Autodesk Inventor part; units mm, degrees
ref_plane "YZ Plane" through (0, 0, 0) normal (1, 0, 0) x (0, 1, 0)
ref_plane "XZ Plane" through (0, 0, 0) normal (0, 1, 0) x (-1, 0, 0)
ref_plane "XY Plane" through (0, 0, 0) normal (0, 0, 1) x (1, 0, 0)
sketch "Sketch1" plane through (0, 0, 0) normal (0, 0, 1) x (1, 0, 0)
  line L0 (-25.5, 10) -> (25.5, 10)
  line L1 (25.5, 10) -> (25.5, -10)
  line L2 (25.5, -10) -> (-25.5, -10)
  line L3 (-25.5, -10) -> (-25.5, 10)
  point P0 (0, 0)
  point P1 (0, 10)
  point P2 (25.5, 0)
  dimension "d0" = 51
  dimension "d1" = 20
extrude "Extrusion1" add sketch "Sketch1" along normal blind 5
sketch "Sketch2" plane through (-25.5, -10, 0) normal (0, -1, 0) x (1, 0, 0)
  line L0 (0, 0) -> (51, 0)
  line L1 (10.5, 0) -> (10.5, -34)
  line L2 (10.5, -34) -> (15.5, -34)
  line L3 (15.5, -34) -> (15.5, 0)
  line L4 (35.5, 0) -> (35.5, -34)
  line L5 (35.5, -34) -> (40.5, -34)
  line L6 (40.5, -34) -> (40.5, 0)
  line L7 (15.5, -34) -> (35.5, -34) construction
  line L8 (0, 0) -> (10.5, -34)
  line L9 (4.1864, 0) -> (10.5, -20.444)
  line L10 (51, 0) -> (40.5, -34)
  line L11 (40.5, -20.444) -> (46.8136, 0)
  point P0 (25.5, 0)
  point P1 (25.5, 0)
  point P2 (25.5, -34)
  dimension "d4" = 20
  dimension "d5" = 5
  dimension "d6" = 5
  dimension "d7" = 34
  dimension "d8" = 4
  dimension "d9" = 4
extrude "Extrusion2" add sketch "Sketch2" against normal up to surface (20 mm away) contours L0 L6 L5 L4 | L0 L9 L1 L8 | L1 L0 L3 L2 | L0 L10 L6 L11
sketch "Sketch3" plane through (10, -10, -34) normal (-1, 0, 0) x (0, 0, 1)
  circle A0 centre (10, 10) radius 2.1
  line L0 (0, 0) -> (0, 20)
  point P0 (34, 10)
  point P1 (0, 10)
  dimension "d12" = 4.2
  dimension "d13" = 10
extrude "Extrusion3" cut sketch "Sketch3" along normal blind 40 and the other way blind 40
sketch "Sketch4" plane through (-25.5, 10, 5) normal (0, 1, 0) x (1, 0, 0)
  line L0 (35.5, 15) -> (15.5, 15)
  line L1 (15.5, 15) -> (15.5, 19)
  line L2 (15.5, 19) -> (35.5, 19)
  line L3 (35.5, 19) -> (35.5, 15)
  line L4 (10.5, 39) -> (15.5, 39)
  point P0 (25.5, 5)
  point P1 (35.5, 5)
  point P2 (15.5, 5)
  dimension "d18" = 20
  dimension "d19" = 4
extrude "Extrusion4" add sketch "Sketch4" against normal blind 5
sketch "Sketch6" plane through (0, 0, 5) normal (0, 0, 1) x (1, 0, 0)
  circle A0 centre (18, 0) radius 2.6
  circle A1 centre (-18, 0) radius 2.6
  point P0 (0, 0)
  dimension "d25" = 5.2
  dimension "d26" = 18
  dimension "d27" = 18
extrude "Extrusion6" cut sketch "Sketch6" against normal blind 5
properties part number "GT2_Holder"
CAD build for the part. Positions are in the model's coordinates, mm. A direction names the side the tool comes from. Round coordinates to 2 decimals unless told otherwise and drop trailing zeros. Loops run counter-clockwise (first coordinate to the right, second up) from the corner with the lowest first, then second, coordinate; pieces in that order, holes last. Notation, with made-up numbers: M 73,0 L 100,0 A24 ccw 100,27 Z; hole C 72,66 d10. An arc over 180 degrees is marked long. One line per question, with ' | ' between items. Start each with the question number.
Item 1: Two-plate mould, pull along Z, no slides. Class faces 4 (the cylindrical face through (20.48, 0.78, 2.54)), 5 (the flat face through (20.324, -0.14, -16.762)), 6 (the flat face through (-18.2, -0.14, -10.08)): pulls with the +Z half, pulls with the -Z half, needs draft (parallel to the pull), parting line crosses it, or undercut.
Item 2: Cut at D-D, the plane x = -20. Write the cut outline in (y, z).
Item 3: Which spindle directions (+Z, -Z, +X, -X, +Y, -Y) get a long thin tool onto all of the face, cutting with end or side? Do faces 1 (the flat face through (18.1, -0.1, -10.4)), 2 (the flat face through (0, 5, -12)), 3 (the cylindrical face through (-15.52, 0.78, 2.54)). Say none if no direction does.
Item 4: Cut at C-C, the plane z = -12.5. Write the cut outline in (x, y).
Item 5: Cut at B-B, the plane x = 17. Write the cut outline in (y, z), plus the area to 3 significant figures.
Item 6: Wall check: line 1 (Z direction, x = -6.5, y = 5.5); line 2 (Y direction, x = -18, z = 3); line 3 (Y direction, x = -12.75, z = -24). Give the ranges that are in metal, low to high.
Item 7: Pin check, flat tips, straight feed: pin 1 Ø5 at (x, y) = (7, -4) entering from -Z; pin 2 Ø4 at (y, z) = (-1, -23.5) entering from -X; pin 3 Ø10 at (y, z) = (-2.5, -24) entering from +X. Stop position of each tip, or through.
Item 8: Cut at A-A, the plane y = 6. Write the cut outline in (x, z).
Responses:
1) face 4: needs draft | face 5: pulls with the -Z half | face 6: undercut
2) outline: M -10,-17.81 L 10,-17.81 L 10,-4.25 L -10,-4.25 Z; M -10,0 L -1.66,0 L -1.66,5 L -10,5 Z; M 1.66,0 L 10,0 L 10,5 L 1.66,5 Z
3) face 1: +Y, -Y | face 2: -Z, -Y | face 3: +Z
4) outline: M -21.64,-10 L -17.45,-10 L -17.45,10 L -21.64,10 Z; M -15,-10 L -10,-10 L -10,5 L 10,5 L 10,-10 L 15,-10 L 15,10 L -15,10 Z; M 17.45,-10 L 21.64,-10 L 21.64,10 L 17.45,10 Z
5) outline: M -10,-27.52 L 10,-27.52 L 10,-13.97 L -10,-13.97 Z; M -10,0 L -2.4,0 L -2.4,5 L -10,5 Z; M 2.4,0 L 10,0 L 10,5 L 2.4,5 Z; hole C 0,-24 d4.2 | area: 333 mm²
6) line 1: z = -14 to -10, 0 to 5 | line 2: y = -10 to -2.6, 2.6 to 10 | line 3: y = -10 to -2.1, 2.1 to 10
7) pin 1: stops at z = 0 | pin 2: stops at x = -18.86 | pin 3: stops at x = 19.63
8) outline: M -25.5,0 L -15,-34 L -10,-34 L -10,-14 L 10,-14 L 10,-34 L 15,-34 L 25.5,0 L 25.5,5 L -25.5,5 Z; hole M -21.31,0 L -15,-20.44 L -15,0 Z; hole M -10,-10 L 10,-10 L 10,0 L -10,0 Z; hole M 15,-20.44 L 21.31,0 L 15,0 Z
